Autodesk Inventor part; units mm, degrees
ref_plane "YZ Plane" through (0, 0, 0) normal (1, 0, 0) x (0, 1, 0)
ref_plane "XZ Plane" through (0, 0, 0) normal (0, 1, 0) x (-1, 0, 0)
ref_plane "XY Plane" through (0, 0, 0) normal (0, 0, 1) x (1, 0, 0)
sketch "スケッチ1" plane through (0, 0, 0) normal (0, 0, 1) x (1, 0, 0)
  arc A0 (-20, 29.9333) -> (20, 29.9333) centre (0, 0) ccw
  line L0 (-20, -80) -> (20, -80)
  line L1 (20, -80) -> (20, 80)
  line L2 (20, 80) -> (-20, 80)
  line L3 (-20, 80) -> (-20, -80)
  line L4 (-20, -80) -> (20, 80) construction
  line L5 (20, -80) -> (-20, 80) construction
  dimension "d0" = 72
  dimension "d1" = 80
  dimension "d2" = 40
extrude "プレート1" add sketch "スケッチ1" along normal blind 2.3 contours L3 A0 | L3 L2 L1 A0 | L1 A0
sketch "スケッチ2" plane through (0, 0, 2.3) normal (0, 0, 1) x (1, 0, 0)
  circle A0 centre (0, 0) radius 31
  point P0 (-28.6403, -11.8632)
  point P1 (-11.8632, -28.6403)
  point P2 (11.8632, -28.6403)
  point P3 (28.6403, -11.8632)
  point P4 (28.6403, 11.8632)
  point P5 (11.8632, 28.6403)
  point P6 (-11.8632, 28.6403)
  point P7 (-28.6403, 11.8632)
  dimension "d5" = 62
  dimension "d8" = 360
  dimension "d34" = 0
hole "穴1" at (-28.6403, 11.8632, 2.3) at (-11.8632, 28.6403, 2.3) at (11.8632, 28.6403, 2.3) at (28.6403, 11.8632, 2.3) at (28.6403, -11.8632, 2.3) at (11.8632, -28.6403, 2.3) at (-11.8632, -28.6403, 2.3) at (-28.6403, -11.8632, 2.3) direction (0, 0, -1) diameter 4.3 end through all
sketch "スケッチ4" plane through (0, 0, 2.3) normal (0, 0, 1) x (1, 0, 0)
  line L0 (10, 50) -> (-10, 50)
  line L1 (-10, 50) -> (-10, 70)
  line L2 (-10, 70) -> (10, 70)
  line L3 (10, 70) -> (10, 50)
  line L4 (10, 50) -> (-10, 70) construction
  line L5 (-10, 50) -> (10, 70) construction
  line L6 (-20, 80) -> (20, 80)
  circle A0 centre (0, 0) radius 72.5
  point P0 (0, 60)
  point P1 (0, 60)
  dimension "d21" = 20
  dimension "d22" = 10
  dimension "d33" = 145
  dimension "d38" = 20
hole "穴2" at (-10, 70, 2.3) at (10, 70, 2.3) at (-10, 50, 2.3) at (10, 50, 2.3) direction (0, 0, -1) diameter 5.3 end through all
fillet "コーナーR2" radius 5 2 edges at (-20, 80, 1.15) (20, 80, 1.15)
sketch "スケッチ5" plane through (0, 0, 2.3) normal (0, 0, 1) x (1, 0, 0)
  circle A0 centre (0, 0) radius 24
  dimension "d35" = 48
extrude "押し出し2" cut sketch "スケッチ5" against normal blind 10
fillet "コーナーR3" radius 20 2 edges at (20, 29.9333, 1.15) (-20, 29.9333, 1.15)
equation "\"d16\" = Thickness"
equation "\"d3\" = Thickness"
equation "\"BendRadius\" = Thickness"
equation "\"BendReliefWidth\" = Thickness"
equation "\"BendReliefDepth\" = 0.5 * Thickness"
equation "\"CornerReliefSize\" = 4 * Thickness"
equation "\"MinimumRemnant\" = 2 * Thickness"
equation "\"TransitionRadius\" = BendRadius"
equation "\"JacobiRadiusSize\" = BendRadius"
equation "\"GapSize\" = Thickness"
properties part number "scara-plate8" material "鋼、炭素鋼"
Model file for the job. Use its own axes, mm. Give positions to 0.01 mm unless a question says otherwise; leave off trailing zeros. Loops run counter-clockwise (first coordinate to the right, second up) from the corner with the lowest first, then second, coordinate; pieces in that order, holes last. Notation, with made-up numbers: (88, -20.5) -> (113, -20.5) arc R17 ccw to (113, -14.5) -> close; hole circle Ø9 at (69, 24.25). An arc over 180 degrees is marked (long way). Use CSV: the item, a comma, the result in double quotes. Start each with the question number.
1) Wall check: line 1 (X direction, y = 70, z = 1.85); line 2 (X direction, y = 68, z = 0.6); line 3 (Y direction, x = -0.5, z = 1.3). Give the ranges that are in metal, low to high.
2) Slice it at D-D on z = 1.8. Give the number of separate pieces and of enclosed holes in the cut face, plus the area to 3 significant figures.
3) Flat gauge pins, fed straight in: pin 1 Ø4 at (x, y) = (28.64, 11.86) entering from +Z; pin 2 Ø7 at (x, y) = (-10, 50) entering from -Z. Where does each tip first touch, or does it go through?
4) Slice it at A-A on y = 70. Give the cut face in (x, z), plus the area to 3 significant figures.
5) Slice it at C-C on x = 2. Give the cut face in (y, z).
6) Mould opens along Y. For faces 1 (the flat face through (20, 57, 1)), 2 (the cylindrical face through (13.77, -29.63, 1.13)), 3 (the cylindrical face through (19, 78, 1)), 4 (the cylindrical face through (1.18, -35.98, 1.13)) say: released by +Y, released by -Y, zero draft, split by the parting line, or undercut.
7) Slice it at B-B on y = 0. Give the cut face in (x, z).
Computed values:
1,line 1,"x = -20 to -12.65, -7.35 to 7.35, 12.65 to 20"
1,line 2,"x = -20 to -11.74, -8.26 to 8.26, 11.74 to 20"
1,line 3,"y = -36 to -23.99, 23.99 to 80"
2,separate pieces,"1"
2,enclosed holes,"13"
2,area,"3,910 mm^2"
3,pin 1,"passes through"
3,pin 2,"stops at z = 0"
4,outline,"(-20, 0) -> (-12.65, 0) -> (-12.65, 2.3) -> (-20, 2.3) -> close; (-7.35, 0) -> (7.35, 0) -> (7.35, 2.3) -> (-7.35, 2.3) -> close; (12.65, 0) -> (20, 0) -> (20, 2.3) -> (12.65, 2.3) -> close"
4,area,"67.6 mm^2"
5,outline,"(-35.94, 0) -> (-23.92, 0) -> (-23.92, 2.3) -> (-35.94, 2.3) -> close; (23.92, 0) -> (80, 0) -> (80, 2.3) -> (23.92, 2.3) -> close"
6,face 1,"zero draft"
6,face 2,"undercut"
6,face 3,"released by +Y"
6,face 4,"split by the parting line"
7,outline,"(-36, 0) -> (-24, 0) -> (-24, 2.3) -> (-36, 2.3) -> close; (24, 0) -> (36, 0) -> (36, 2.3) -> (24, 2.3) -> close"
